Input: part model. Units: mm. Frame: model coordinates. A direction names the side the tool comes from. Give positions to 0.01 mm unless a question says otherwise; leave off trailing zeros. Loops run counter-clockwise (first coordinate to the right, second up) from the corner with the lowest first, then second, coordinate; pieces in that order, holes last. Notation, with made-up numbers: M 52,23 L 97,23 A26 cw 97,54 Z; hole C -20.5,3 d3. An arc over 180 degrees is marked long. Use a Markdown table: item, result. Add a question column.
from build123d import *

# Parameters (mm, degrees)
F0_W      = 609.6
F0_H      = 609.6
F1_DEPTH  = 238.125
F3_DEPTH  = 609.601
F4_W      = 76.2
F4_H      = 542.925
F5_DEPTH  = 476.251
F6_R      = 191.690625
F7_DEPTH  = 12.7
F9_D      = 25.4
F9_DEPTH  = 34.925
F9_TIP    = 7.6309298617
F10_W     = 346.075
F10_H     = 279.4
F11_DEPTH = 4.7625


# Not quite as in the source:
# - a pattern or mirror of a feature is missing from the dataset's text; its kind, count and spacing are read off the source's solid


with BuildPart() as f1:
    # F0 (on Top) → F1 (new body, symmetric)
    with BuildSketch(Plane.XY):
        Rectangle(F0_W, F0_H)
    extrude(amount=F1_DEPTH, both=True)

    # F2 (on face) → F3 (cut, through all)
    with BuildSketch(Plane.XZ.offset(304.8)):
        with BuildLine():
            ThreePointArc((-193.9860043921, -100.965), (-230.9234761066, -170.6305134371), (-243.68125, -248.44375))
            Line((-243.68125, -248.44375), (243.68125, -248.44375))
            ThreePointArc((243.68125, -248.44375), (230.9234761066, -170.6305134371), (193.9860043921, -100.965))
            ThreePointArc((193.9860043921, -100.965), (0, -3.175), (-193.9860043921, -100.965))
        make_face()
    extrude(amount=-F3_DEPTH, mode=Mode.SUBTRACT)

    # F4 (on face) → F5 (cut, through all)
    with BuildSketch(Plane.XY.offset(238.125)):
        with Locations((304.8, 0)):
            Rectangle(F4_W, F4_H)
        with Locations((-304.8, 0)):
            Rectangle(F4_W, F4_H)
    extrude(amount=-F5_DEPTH, mode=Mode.SUBTRACT)

    # F6 (on face) → F7 (join)
    with BuildSketch(Plane.XY.offset(238.125)):
        with BuildLine():
            ThreePointArc((-231.775, -136.128125), (-211.4711543972, -108.732394395), (-179.3535020392, -120.1878999995))
            ThreePointArc((-179.3535020392, -120.1878999995), (0, -215.9), (179.3535020392, -120.1878999995))
            ThreePointArc((179.3535020392, -120.1878999995), (211.4711543972, -108.732394395), (231.775, -136.128125))
            Line((231.775, -136.128125), (231.775, -247.65))
            Line((231.775, -247.65), (266.7, -247.65))
            Line((266.7, -247.65), (266.7, 247.65))
            Line((266.7, 247.65), (231.775, 247.65))
            Line((231.775, 247.65), (231.775, 136.128125))
            ThreePointArc((231.775, 136.128125), (211.4711543972, 108.732394395), (179.3535020392, 120.1878999995))
            ThreePointArc((179.3535020392, 120.1878999995), (0, 215.9), (-179.3535020392, 120.1878999995))
            ThreePointArc((-179.3535020392, 120.1878999995), (-211.4711543972, 108.732394395), (-231.775, 136.128125))
            Line((-231.775, 136.128125), (-231.775, 247.65))
            Line((-231.775, 247.65), (-266.7, 247.65))
            Line((-266.7, 247.65), (-266.7, -247.65))
            Line((-266.7, -247.65), (-231.775, -247.65))
            Line((-231.775, -247.65), (-231.775, -136.128125))
        make_face()
        Circle(F6_R, mode=Mode.SUBTRACT)
    extrude(amount=F7_DEPTH)

    # F9
    with Locations(Plane.XY.offset(238.125)):
        with Locations((0, 0)):
            Hole(F9_D / 2, depth=F9_DEPTH)
            with Locations((0, 0, -(F9_DEPTH + F9_TIP / 2))):  # 118° drill point
                Cone(0, F9_D / 2, F9_TIP, mode=Mode.SUBTRACT)

    # F10 (on face) → F11 (cut)
    with BuildSketch(Plane.YZ.offset(266.7)):
        with BuildLine():
            Line((179.3875, -117.475), (244.475, -117.475))
            ThreePointArc((244.475, -117.475), (247.65, -114.3), (244.475, -111.125))
            Line((244.475, -111.125), (179.3875, -111.125))
            Line((179.3875, -111.125), (179.3875, 168.275))
            Line((179.3875, 168.275), (244.475, 168.275))
            ThreePointArc((244.475, 168.275), (247.65, 171.45), (244.475, 174.625))
            Line((244.475, 174.625), (179.3875, 174.625))
            Line((179.3875, 174.625), (179.3875, 206.375))
            ThreePointArc((179.3875, 206.375), (176.2125, 209.55), (173.0375, 206.375))
            Line((173.0375, 206.375), (173.0375, 174.625))
            Line((173.0375, 174.625), (-173.0375, 174.625))
            Line((-173.0375, 174.625), (-173.0375, 206.375))
            ThreePointArc((-173.0375, 206.375), (-176.2125, 209.55), (-179.3875, 206.375))
            Line((-179.3875, 206.375), (-179.3875, 174.625))
            Line((-179.3875, 174.625), (-244.475, 174.625))
            ThreePointArc((-244.475, 174.625), (-247.65, 171.45), (-244.475, 168.275))
            Line((-244.475, 168.275), (-179.3875, 168.275))
            Line((-179.3875, 168.275), (-179.3875, -111.125))
            Line((-179.3875, -111.125), (-244.475, -111.125))
            ThreePointArc((-244.475, -111.125), (-247.65, -114.3), (-244.475, -117.475))
            Line((-244.475, -117.475), (-179.3875, -117.475))
            Line((-179.3875, -117.475), (-179.3875, -187.325))
            ThreePointArc((-179.3875, -187.325), (-176.2125, -190.5), (-173.0375, -187.325))
            Line((-173.0375, -187.325), (-173.0375, -117.475))
            Line((-173.0375, -117.475), (173.0375, -117.475))
            Line((173.0375, -117.475), (173.0375, -187.325))
            ThreePointArc((173.0375, -187.325), (176.2125, -190.5), (179.3875, -187.325))
            Line((179.3875, -187.325), (179.3875, -117.475))
        make_face()
        with Locations((0, 28.575)):
            Rectangle(F10_W, F10_H, mode=Mode.SUBTRACT)
    f11 = extrude(amount=-F11_DEPTH, mode=Mode.SUBTRACT)

    # F11_copies: F11 across plane
    add(f11.mirror(Plane(origin=(0, 0, 0), x_dir=(0, 0, -1), z_dir=(-1, 0, 0))), mode=Mode.SUBTRACT)


solid = f1.part
1) Section query B-B, the plane y = -257.5. Return the cut outline in (x, z) (1 decimal), and give its area (3 significant figures).
2) Section query C-C, the plane x = -222.5. Return the cut outline in (y, z) (3 decimals).
3) Ray query, line 1 (Z direction, x = 266, y = 115.5) (3 decimals); line 2 (Y direction, x = 0, z = 224); line 3 (X direction, y = 263, z = 18). Return the intervals inside material, ascending. Write a range as [from, to].
4) Pull-direction query (X, two-part tool) for faces 1 (the cylindrical face through (-228.87, -4.27, -164.78)), 2 (the flat face through (-286, 271.462, 3)), 3 (the flat face through (304.8, 288, 3)); classes: pulls with the +X half, pulls with the -X half, needs draft (parallel to the pull), parting line crosses it, or undercut.
5) Section query D-D, the plane z = 77.5. Return the cut outline in (x, y).
6) Reachability of faces 4 (the cylindrical face through (-2.96, -215.88, 244.39)), 5 (the cylindrical face through (229.573, -4.267, -166.733)), 6 (the flat face through (266.7, -4, -153)), 7 (the flat face through (-266.7, -2, 31)), 8 (the cylindrical face through (212, 108.9, 244.4)) from +Z, -Z, +X, -X, +Y, -Y: full face, straight path, thin tool, end or side. Return the list, or none.
7) Contact query for flat-ended pins moving along their axis: P1, Ø2, axis at x = -68, y = -222.5, coming from the -Z side; P2, Ø12, axis at y = 4, z = 27, coming from the -X side; P3, Ø20.5, axis at x = 0, y = 0, coming from the +Z side. Output: stop coordinate, or through.
Entries:
| question | item | result |
|---|---|---|
| 1 | outline | M -266.7,-238.1 L -243.5,-238.1 A243.7 cw -194,-101 A241.3 cw 194,-101 A243.7 cw 243.5,-238.1 L 266.7,-238.1 L 266.7,238.1 L -266.7,238.1 Z |
| 1 | area | 165,000 mm² |
| 2 | outline | M -304.8,-149.074 L 304.8,-149.074 L 304.8,238.125 L 115.03,238.125 L 115.03,250.825 L -115.03,250.825 L -115.03,238.125 L -304.8,238.125 Z |
| 3 | line 1 | z = [-238.125, -117.475], [-111.125, 168.275], [174.625, 250.825] |
| 3 | line 2 | y = [-304.8, -12.7], [12.7, 304.8] |
| 3 | line 3 | x = [-266.7, 266.7] |
| 4 | face 1 | undercut |
| 4 | face 2 | needs draft |
| 4 | face 3 | pulls with the +X half |
| 5 | outline | M -304.8,-304.8 L 304.8,-304.8 L 304.8,-271.46 L 266.7,-271.46 L 266.7,-179.39 L 261.94,-179.39 L 261.94,-173.04 L 266.7,-173.04 L 266.7,173.04 L 261.94,173.04 L 261.94,179.39 L 266.7,179.39 L 266.7,271.46 L 304.8,271.46 L 304.8,304.8 L -304.8,304.8 L -304.8,271.46 L -266.7,271.46 L -266.7,179.39 L -261.94,179.39 L -261.94,173.04 L -266.7,173.04 L -266.7,-173.04 L -261.94,-173.04 L -261.94,-179.39 L -266.7,-179.39 L -266.7,-271.46 L -304.8,-271.46 Z |
| 6 | face 4 | +Z, -Y |
| 6 | face 5 | -Z, +Y, -Y |
| 6 | face 6 | +Z, -Z, +X |
| 6 | face 7 | +Z, -Z, -X |
| 6 | face 8 | +Z, +Y |
| 7 | P1 | stops at z = -13.25 |
| 7 | P2 | stops at x = -266.7 |
| 7 | P3 | stops at z = 201.73 |
